Part model, mm, in its own coordinate system. A direction names the side the tool comes from. Round coordinates to 2 decimals unless told otherwise and drop trailing zeros. Loops run counter-clockwise (first coordinate to the right, second up) from the corner with the lowest first, then second, coordinate; pieces in that order, holes last. Notation, with made-up numbers: (-4, 11) - (18, 11) arc R10 cw to (18, 27) - close; hole circle Ø3 at (-19.5, -16). An arc over 180 degrees is marked (long way). Put each result on its own line as item: value.
from build123d import *

# Parameters (mm, degrees)
SKETCH1_R           = 4.9
SKETCH1_R_2         = 1.65
BOSS_EXTRUDE1_DEPTH = 2.3
FILLET1_R           = 3
SKETCH3_R           = 2.75
SKETCH3_R_2         = 0.975
BOSS_EXTRUDE2_DEPTH = 6
CUT_EXTRUDE1_DEPTH  = 2.3
SKETCH5_R           = 7
SKETCH5_R_2         = 4.9
BOSS_EXTRUDE3_DEPTH = 4.5
BOSS_EXTRUDE4_START = 6
SKETCH6_R           = 2
BOSS_EXTRUDE4_DEPTH = 2
BOSS_EXTRUDE5_START = -6
SKETCH6_2_R         = 2
BOSS_EXTRUDE5_DEPTH = 2
SKETCH7_R           = 0.104776465
SKETCH7_R_2         = 0.95
CUT_EXTRUDE2_DEPTH  = 16
SKETCH8_R           = 2
CUT_EXTRUDE3_DEPTH  = 2.3
SKETCH10_R          = 2
SKETCH10_R_2        = 1.65
BOSS_EXTRUDE8_DEPTH = 1


with BuildPart() as part:
    # Sketch1 → Boss-Extrude1 (new body)
    with BuildSketch(Plane(origin=(0, 0, 0), x_dir=(1, 0, 0), z_dir=(0, 1, 0))):
        with BuildLine():
            Line((-19.311278394, 3.635335273), (-15, 6.402726073))
            Line((-15, 6.402726073), (-15, 12))
            Line((-15, 12), (15, 12))
            Line((15, 12), (15, 6.97678585))
            Line((15, 6.97678585), (20, 3.7))
            ThreePointArc((20, 3.7), (23.7, 0), (20, -3.7))
            Line((20, -3.7), (15, -6.97678585))
            Line((15, -6.97678585), (15, -12))
            Line((15, -12), (-15, -12))
            Line((-15, -12), (-15, -6.402726073))
            Line((-15, -6.402726073), (-19.311278394, -3.635335273))
            ThreePointArc((-19.311278394, -3.635335273), (-23.7, 0), (-19.311278394, 3.635335273))
        make_face()
        Circle(SKETCH1_R, mode=Mode.SUBTRACT)
        with Locations((-20, 0)):
            Circle(SKETCH1_R_2, mode=Mode.SUBTRACT)
        with Locations((20, 0)):
            Circle(SKETCH1_R_2, mode=Mode.SUBTRACT)
    extrude(amount=BOSS_EXTRUDE1_DEPTH)

    # Fillet1
    fillet1_edges = [part.edges().sort_by_distance(p)[0] for p in [
        (-15, 1.15, -12),
        (15, 1.15, -12),
        (15, 1.15, 12),
        (-15, 1.15, 12),
    ]]
    fillet(fillet1_edges, radius=FILLET1_R)

    # Sketch3 → Boss-Extrude2 (add)
    with BuildSketch(Plane(origin=(0, 2.3, 0), x_dir=(1, 0, 0), z_dir=(0, 1, 0))):
        with Locations((-12, 9)):
            Circle(SKETCH3_R)
        with Locations((-12, 9)):
            Circle(SKETCH3_R_2, mode=Mode.SUBTRACT)
        with Locations((12, 9)):
            Circle(SKETCH3_R)
        with Locations((12, 9)):
            Circle(SKETCH3_R_2, mode=Mode.SUBTRACT)
        with Locations((12, -9)):
            Circle(SKETCH3_R)
        with Locations((12, -9)):
            Circle(SKETCH3_R_2, mode=Mode.SUBTRACT)
        with Locations((-12, -9)):
            Circle(SKETCH3_R)
        with Locations((-12, -9)):
            Circle(SKETCH3_R_2, mode=Mode.SUBTRACT)
    extrude(amount=BOSS_EXTRUDE2_DEPTH)

    # Sketch4 → Cut-Extrude1 (cut)
    with BuildSketch(Plane(origin=(0, 2.3, 0), x_dir=(1, 0, 0), z_dir=(0, 1, 0))):
        with BuildLine():
            Line((-12, 12), (-12, 16.294257714))
            Line((-12, 16.294257714), (12, 16.294257714))
            Line((12, 16.294257714), (12, 15.219911052))
            Line((12, 15.219911052), (12, 12))
            add(Edge.make_bspline(
                [(-12, 12), (-9.057245707, 12), (-4.223972764, 9.428637942), (3.764574149, 9.238075055), (9.81416723, 12), (12, 12)],
                knots=[0, 0, 0, 0, 0.370531455, 0.610499762, 1, 1, 1, 1], degree=3))
        make_face()
        with BuildLine():
            Line((12, -16.294257714), (12, -15.219911052))
            Line((12, -15.219911052), (12, -12))
            add(Edge.make_bspline(
                [(-12, -12), (-9.057245707, -12), (-4.223972764, -9.428637942), (3.764574149, -9.238075055), (9.81416723, -12), (12, -12)],
                knots=[0, 0, 0, 0, 0.370531455, 0.610499762, 1, 1, 1, 1], degree=3))
            Line((-12, -12), (-12, -16.294257714))
            Line((-12, -16.294257714), (12, -16.294257714))
        make_face()
    extrude(amount=-CUT_EXTRUDE1_DEPTH, mode=Mode.SUBTRACT)

    # Sketch5 → Boss-Extrude3 (add)
    with BuildSketch(Plane(origin=(0, 2.3, 0), x_dir=(1, 0, 0), z_dir=(0, 1, 0))):
        Circle(SKETCH5_R)
        Circle(SKETCH5_R_2, mode=Mode.SUBTRACT)
    extrude(amount=BOSS_EXTRUDE3_DEPTH)

    # Sketch6 → Boss-Extrude4 (add)
    with BuildSketch(Plane(origin=(0, 0, 0), x_dir=(0, 0, -1), z_dir=(1, 0, 0)).offset(BOSS_EXTRUDE4_START)):
        with Locations((0, 4.55)):
            Circle(SKETCH6_R)
    extrude(amount=BOSS_EXTRUDE4_DEPTH)

    # Sketch6<2> → Boss-Extrude5 (add)
    with BuildSketch(Plane(origin=(0, 0, 0), x_dir=(0, 0, -1), z_dir=(1, 0, 0)).offset(BOSS_EXTRUDE5_START)):
        with Locations((0, 4.55)):
            Circle(SKETCH6_2_R)
    extrude(amount=-BOSS_EXTRUDE5_DEPTH)

    # Sketch7 → Cut-Extrude2 (cut)
    with BuildSketch(Plane(origin=(8, 0, 0), x_dir=(0, 0, -1), z_dir=(1, 0, 0))):
        with Locations((-18.077789398, 8.361547887)):
            Circle(SKETCH7_R)
        with Locations((0, 4.55)):
            Circle(SKETCH7_R_2)
    extrude(amount=-CUT_EXTRUDE2_DEPTH, mode=Mode.SUBTRACT)

    # Sketch8 → Cut-Extrude3 (cut)
    with BuildSketch(Plane(origin=(0, 2.3, 0), x_dir=(1, 0, 0), z_dir=(0, 1, 0))):
        with Locations((-14.5, 0)):
            Circle(SKETCH8_R)
        with Locations((14.5, 0)):
            Circle(SKETCH8_R)
    extrude(amount=-CUT_EXTRUDE3_DEPTH, mode=Mode.SUBTRACT)

    # Sketch10 → Boss-Extrude8 (add)
    with BuildSketch(Plane.XZ):
        with BuildLine():
            Line((-20, 3.63), (-14.5, 3.63))
            ThreePointArc((-14.5, 3.63), (-10.87, 0), (-14.5, -3.63))
            Line((-14.5, -3.63), (-20, -3.63))
            ThreePointArc((-20, -3.63), (-23.63, 0), (-20, 3.63))
        make_face()
        with Locations((-14.5, 0)):
            Circle(SKETCH10_R, mode=Mode.SUBTRACT)
        with Locations((-20, 0)):
            Circle(SKETCH10_R_2, mode=Mode.SUBTRACT)
        with BuildLine():
            Line((14.5, 3.63), (20, 3.63))
            ThreePointArc((20, 3.63), (23.63, 0), (20, -3.63))
            Line((20, -3.63), (14.5, -3.63))
            ThreePointArc((14.5, -3.63), (10.87, 0), (14.5, 3.63))
        make_face()
        with Locations((14.5, 0)):
            Circle(SKETCH10_R, mode=Mode.SUBTRACT)
        with Locations((20, 0)):
            Circle(SKETCH10_R_2, mode=Mode.SUBTRACT)
    extrude(amount=BOSS_EXTRUDE8_DEPTH)


solid = part.part
1. Band-saw the part on A-A (x = 14). List the corners of the cut face in (y, z), plus the area to 3 significant figures.
A:
outline: (-1, -3.6) - (0, -3.6) - (0, -11.24) - (2.3, -11.24) - (2.3, -10.89) - (8.3, -10.89) - (8.3, -7.11) - (2.3, -7.11) - (2.3, -1.94) - (-1, -1.94) - close; (-1, 1.94) - (2.3, 1.94) - (2.3, 7.11) - (8.3, 7.11) - (8.3, 10.89) - (2.3, 10.89) - (2.3, 11.24) - (0, 11.24) - (0, 3.6) - (-1, 3.6) - close
area: 91.4 mm²
2. Pin check, flat tips, straight feed: P1, Ø5, axis at y = 5, z = -0.5, coming from the +X side; P2, Ø5, axis at y = 5, z = -7, coming from the +X side; P3, Ø1, axis at x = -5.5, y = 3, coming from the +Z side. Stop position of each tip, or through.
A:
P1: stops at x = 8
P2: stops at x = 14.75
P3: stops at z = 4.9
3. Tool access for faces 1 (the flat face through (15, 1, -8)), 2 (the flat face through (-17.2, -0.5, -3.63)), 3 (the cylindrical face through (14.62, 5.26, -9.83)), 4 (the flat face through (-15, 1, 8)): list every direction of +Z, -Z, +X, -X, +Y, -Y with a clear straight run to the whole face (end or side of a thin tool).
A:
face 1: -Z, +X, +Y, -Y
face 2: -Z, +X, -X, -Y
face 3: +Y
face 4: +Z, -X, +Y, -Y
4. Band-saw the part on C-C (z = 7.5). List the corners of the cut face in (x, y), plus the area to 3 significant figures.
A:
outline: (-15, 0) - (15, 0) - (15, 2.3) - (14.3, 2.3) - (14.3, 8.3) - (9.7, 8.3) - (9.7, 2.3) - (-9.7, 2.3) - (-9.7, 8.3) - (-14.3, 8.3) - (-14.3, 2.3) - (-15, 2.3) - close
area: 124 mm²
5. Probe line 1 along X through (y, z) = (1.55, 0); line 2 along X through (y, z) = (-0.65, 0); line 3 along Z through (x, y) = (-12, 5.5) (3 decimals). List the from-to ranges inside material, lowest first. Write a range as [from, to].
A:
line 1: x = [-23.7, -21.65], [-18.35, -16.5], [-12.5, -4.9], [4.9, 12.5], [16.5, 18.35], [21.65, 23.7]
line 2: x = [-23.63, -21.65], [-18.35, -16.5], [-12.5, -10.87], [10.87, 12.5], [16.5, 18.35], [21.65, 23.63]
line 3: z = [-11.75, -9.975], [-8.025, -6.25], [6.25, 8.025], [9.975, 11.75]
6. Two-plate mould, pull along X, no slides. Class faces 5 (the flat face through (12, 2.3, 9)), 6 (the cylindrical face through (14.1, 1.17, 11.14)), 7 (the cylindrical face through (-6.381, 5.492, 0.124)), 8 (the cylindrical face through (-9.38, 5.26, -9.83)): pulls with the +X half, pulls with the -X half, needs draft (parallel to the pull), parting line crosses it, or undercut.
A:
face 5: undercut
face 6: pulls with the +X half
face 7: needs draft
face 8: undercut
7. Band-saw the part on B-B (z = 0). Give the number of separate pieces and of enclosed holes in the cut face, plus the area to 3 significant figures.
A:
separate pieces: 8
enclosed holes: 0
area: 78.9 mm²
